Could you check a few things on this model? Use its own coordinates, in mm. Face numbers are marked on the shaded views. A direction names the side the tool comes from. Coordinates: 2 decimals unless noted, no trailing zeros. Write each loop counter-clockwise with the first axis right and the second up, starting at its lowest first coordinate (ties: lowest second). Pieces come first, ordered by that corner, then holes. Notation, with made-up numbers: M 78,11 L 107,11 A30 cw 107,38 Z; hole C -23.5,13 d5. An arc over 180 degrees is marked long. Write item = value, one per line.
```python
from build123d import *

# Parameters (mm, degrees)
SKETCH1_R           = 8.5
BOSS_EXTRUDE1_DEPTH = 5.8
SKETCH2_R           = 8
CUT_EXTRUDE1_DEPTH  = 3.2
SKETCH3_R           = 1
BOSS_EXTRUDE2_DEPTH = 3.2
CHAMFER1_SIZE       = 2.65
CHAMFER1_SIZE2      = 3.048476279
SKETCH4_R           = 2.1
BOSS_EXTRUDE3_DEPTH = 3
SKETCH5_R           = 0.85
CUT_EXTRUDE2_DEPTH  = 40.372371259
SKETCH6_R           = 1.1
CUT_EXTRUDE3_DEPTH  = 3


with BuildPart() as part:
    # Sketch1 → Boss-Extrude1 (new body)
    with BuildSketch(Plane.XY):
        with Locations((-29.082250471, -1.703826149)):
            Circle(SKETCH1_R)
    extrude(amount=BOSS_EXTRUDE1_DEPTH)

    # Sketch2 → Cut-Extrude1 (cut)
    with BuildSketch(Plane(origin=(0, 0, 0), x_dir=(-1, 0, 0), z_dir=(0, 0, -1))):
        with Locations((29.082250471, -1.703826149)):
            Circle(SKETCH2_R)
    extrude(amount=-CUT_EXTRUDE1_DEPTH, mode=Mode.SUBTRACT)

    # Sketch3 → Boss-Extrude2 (add)
    with BuildSketch(Plane(origin=(0, 0, 3.2), x_dir=(-1, 0, 0), z_dir=(0, 0, -1))):
        with Locations((29.082250471, -1.703826149)):
            Circle(SKETCH3_R)
    extrude(amount=BOSS_EXTRUDE2_DEPTH)

    # Chamfer1
    chamfer1_edges = [part.edges().sort_by_distance(p)[0] for p in [
        (-28.082250471, -1.703826149, 3.2),
    ]]
    chamfer1_side = [part.faces().sort_by_distance(p)[0] for p in [
        (-21.308524641, -1.703826149, 3.2),
    ]]
    chamfer(chamfer1_edges, length=CHAMFER1_SIZE, length2=CHAMFER1_SIZE2, reference=chamfer1_side[0])

    # Sketch4 → Boss-Extrude3 (add)
    with BuildSketch(Plane(origin=(0, 0, 0), x_dir=(-1, 0, 0), z_dir=(0, 0, -1))):
        with Locations((29.082250471, -1.703826149)):
            Circle(SKETCH4_R)
    extrude(amount=-BOSS_EXTRUDE3_DEPTH)

    # Sketch5 → Cut-Extrude2 (cut, through all)
    with BuildSketch(Plane(origin=(0, 0, 0), x_dir=(-1, 0, 0), z_dir=(0, 0, -1))):
        with Locations((29.082250471, -1.703826149)):
            Circle(SKETCH5_R)
    extrude(amount=-CUT_EXTRUDE2_DEPTH, mode=Mode.SUBTRACT)

    # Sketch6 → Cut-Extrude3 (cut)
    with BuildSketch(Plane.XY.offset(5.8)):
        with Locations((-29.082250471, -1.703826149)):
            Circle(SKETCH6_R)
    extrude(amount=-CUT_EXTRUDE3_DEPTH, mode=Mode.SUBTRACT)


solid = part.part
```
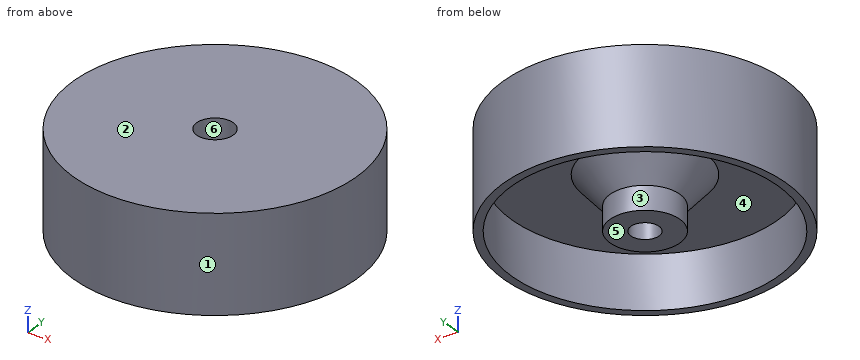
Item 1: Imagine slicing it at A-A (z = 1.05). Write out the boundary of the cut face in (x, y).
Numbers:
outline = C -29.08,-1.7 d17; C -29.08,-1.7 d4.2; hole C -29.08,-1.7 d16; hole C -29.08,-1.7 d1.7
Item 2: For the marked faces 4, 5 and 6, which set-ups out of +Z, -Z, +X, -X, +Y, -Y let a thin tool reach every point of the face, with its end or its side?
Numbers:
face_4 = -Z
face_5 = -Z, +X, -X, +Y, -Y
face_6 = +Z
Item 3: If I drill on line 1 along X through (y, z) = (-4.5, 3); line 2 along Y through (x, z) = (-30.5, 1.2); line 3 along X through (y, z) = (-2.25, 1.4), over which ranges is the centre line in solid material (lowest first)?
Numbers:
line_1 = -37.11 to -36.58, -31.15 to -27.02, -21.59 to -21.06
line_2 = -10.08 to -9.58, -3.25 to -0.15, 6.17 to 6.68
line_3 = -37.56 to -37.06, -31.11 to -29.73, -28.43 to -27.05, -21.1 to -20.6
Item 4: If we mould it in two halves opening along X, with no side actions, what happens to the marked faces 1, 2 and 3? For each: pulls with the +X half, pulls with the -X half, needs draft (parallel to the pull), parting line crosses it, or undercut.
Numbers:
face_1 = parting line crosses it
face_2 = needs draft
face_3 = undercut
Item 5: Imagine slicing it at B-B (y = -8.25). Write out the boundary of the cut face in (x, z).
Numbers:
outline = M -34.5,0 L -33.68,0 L -33.68,3.2 L -24.48,3.2 L -24.48,0 L -23.66,0 L -23.66,5.8 L -34.5,5.8 Z
Item 6: I'm going to push flat-ended pins straight in: P1, Ø2, axis at x = -25.5, z = 3, coming from the +Y side; P2, Ø1, axis at y = -3, z = 2, coming from the +X side; P3, Ø1, axis at x = -22.5, y = -4.5, coming from the -Z side. Where does each tip first touch, or does it pass through?
Numbers:
P1 = 6.39
P2 = -20.62
P3 = 3.2
Item 7: Imagine slicing it at C-C (x = -23.75). Write out the boundary of the cut face in (y, z), and give its area (3 significant figures).
Numbers:
outline = M -8.32,0 L -7.67,0 L -7.67,3.2 L 4.26,3.2 L 4.26,0 L 4.92,0 L 4.92,5.8 L -8.32,5.8 Z
area = 38.6 mm²
Item 8: Imagine slicing it at D-D (z = 3.75). Write out the boundary of the cut face in (x, y), and give its area (3 significant figures).
Numbers:
outline = C -29.08,-1.7 d17; hole C -29.08,-1.7 d2.2
area = 223 mm²
